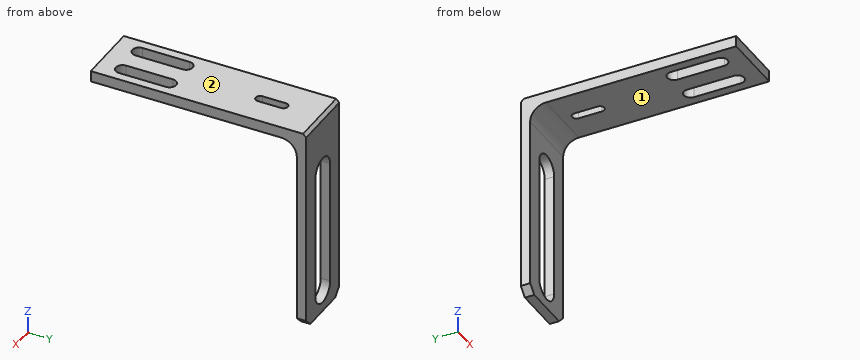
```python
from build123d import *

# Parameters (mm, degrees)
SKETCH2_W           = 40
SKETCH2_H           = 137.5
BOSS_EXTRUDE1_DEPTH = 7
SKETCH4_W           = 40
SKETCH4_H           = 125
BOSS_EXTRUDE2_DEPTH = 6
FILLET1_R           = 10
CHAMFER1_SIZE       = 5
CHAMFER2_SIZE       = 2


with BuildPart() as part:
    # Sketch2 → Boss-Extrude1 (new body)
    with BuildSketch(Plane.XY):
        with Locations((0, 33.75)):
            Rectangle(SKETCH2_W, SKETCH2_H)
        with BuildLine():
            Line((-5.75, 10), (-5.75, -20))
            ThreePointArc((-5.75, -20), (-10, -24.25), (-14.25, -20))
            Line((-14.25, -20), (-14.25, 10))
            ThreePointArc((-14.25, 10), (-10, 14.25), (-5.75, 10))
        make_face(mode=Mode.SUBTRACT)
        with BuildLine():
            Line((5.75, 10), (5.75, -20))
            ThreePointArc((5.75, -20), (10, -24.25), (14.25, -20))
            Line((14.25, -20), (14.25, 10))
            ThreePointArc((14.25, 10), (10, 14.25), (5.75, 10))
        make_face(mode=Mode.SUBTRACT)
        with BuildLine():
            Line((2.75, 77.5), (2.75, 62.5))
            ThreePointArc((2.75, 62.5), (0, 59.75), (-2.75, 62.5))
            Line((-2.75, 62.5), (-2.75, 77.5))
            ThreePointArc((-2.75, 77.5), (0, 80.25), (2.75, 77.5))
        make_face(mode=Mode.SUBTRACT)
    extrude(amount=BOSS_EXTRUDE1_DEPTH)

    # Sketch4 → Boss-Extrude2 (add)
    with BuildSketch(Plane(origin=(0, 102.5, 0), x_dir=(1, 0, 0), z_dir=(0, 1, 0))):
        with Locations((0, 62.5)):
            Rectangle(SKETCH4_W, SKETCH4_H)
        with BuildLine():
            Line((-9, 30), (-9, 110))
            ThreePointArc((-9, 110), (0, 119), (9, 110))
            Line((9, 110), (9, 30))
            ThreePointArc((9, 30), (0, 21), (-9, 30))
        make_face(mode=Mode.SUBTRACT)
    extrude(amount=-BOSS_EXTRUDE2_DEPTH)

    # Fillet1
    fillet1_edges = [part.edges().sort_by_distance(p)[0] for p in [
        (0, 96.5, 0),
    ]]
    fillet(fillet1_edges, radius=FILLET1_R)

    # Chamfer1
    chamfer1_edges = [part.edges().sort_by_distance(p)[0] for p in [
        (-20, 99.5, -125),
        (20, 99.5, -125),
    ]]
    chamfer(chamfer1_edges, length=CHAMFER1_SIZE)

    # Chamfer2
    chamfer2_edges = [part.edges().sort_by_distance(p)[0] for p in [
        (0, 102.5, 7),
    ]]
    chamfer(chamfer2_edges, length=CHAMFER2_SIZE)


solid = part.part
```
Geometry check sheet. Reference: the model listing, model coordinates, mm. Face numbers are marked on the shaded views. A direction names the side the tool comes from. Give positions to 0.01 mm unless a question says otherwise; leave off trailing zeros. Order: outer loops, then holes, each group sorted by start corner. A loop starts at its lowest first (then second) coordinate and runs counter-clockwise, first axis right, second up. Notation, with made-up numbers: (-19, -12.75) - (-4, -12.75) arc R6 cw to (-4, -4.75) - close; hole circle Ø8 at (53, 52). An arc over 180 degrees is marked (long way). Answer in a Markdown table with one row per item. Add a question column.
Q1. Material ranges on probe 1 along Y at (x, z) = (-9.5, -103); probe 2 along Z at (x, y) = (13, 48); probe 3 along Y at (x, z) = (2.5, -4.5), recorded low to high. Write a range as from..to.
Q2. Cross-section at D-D, the plane x = 17.5. Enter the section's corners in (y, z), then the cut area to 3 significant figures.
Q3. Tool access check on the marked faces 1 and 2. Record the directions out of +Z, -Z, +X, -X, +Y, -Y that give a thin tool (end or side, any length) a straight path to the whole face; none if there is none.
Q4. Cross-section at A-A, the plane y = -5. Enter the section's corners in (x, z), then the cut area to 3 significant figures.
Q5. Gauge pin test, flat ends, axial feed: pin 1 (3 mm diameter, centred on x = -15, y = 56.5, fed in from -Z); pin 2 (20 mm diameter, centred on x = -8, z = -74.5, fed in from -Y). Record the tip position at first contact, or that the pin passes through.
Q6. Cross-section at B-B, the plane x = 0. Enter the section's corners in (y, z).
Q7. Cross-section at C-C, the plane z = -86. Enter the section's corners in (x, y).
Check values:
| question | item | result |
|---|---|---|
| 1 | probe 1 | y = 96.5..102.5 |
| 1 | probe 2 | z = 0..7 |
| 1 | probe 3 | y = 94.85..102.5 |
| 2 | outline | (-35, 0) - (86.5, 0) arc R10 cw to (96.5, -10) - (96.5, -122.5) - (102.5, -122.5) - (102.5, 5) - (100.5, 7) - (-35, 7) - close |
| 2 | area | 1,720 mm^2 |
| 3 | face 1 | -Z, +X, -X, -Y |
| 3 | face 2 | +Z, +X, -X, +Y, -Y |
| 4 | outline | (-20, 0) - (-14.25, 0) - (-14.25, 7) - (-20, 7) - close; (-5.75, 0) - (5.75, 0) - (5.75, 7) - (-5.75, 7) - close; (14.25, 0) - (20, 0) - (20, 7) - (14.25, 7) - close |
| 4 | area | 161 mm^2 |
| 5 | pin 1 | stops at z = 0 |
| 5 | pin 2 | stops at y = 96.5 |
| 6 | outline | (-35, 0) - (59.75, 0) - (59.75, 7) - (-35, 7) - close; (80.25, 0) - (86.5, 0) arc R10 cw to (96.5, -10) - (96.5, -21) - (102.5, -21) - (102.5, 5) - (100.5, 7) - (80.25, 7) - close; (96.5, -125) - (102.5, -125) - (102.5, -119) - (96.5, -119) - close |
| 7 | outline | (-20, 96.5) - (-9, 96.5) - (-9, 102.5) - (-20, 102.5) - close; (9, 96.5) - (20, 96.5) - (20, 102.5) - (9, 102.5) - close |
